Input: part model. Units: mm. Frame: model coordinates. A direction names the side the tool comes from. Coordinates: 2 decimals unless noted, no trailing zeros. Write each loop counter-clockwise with the first axis right and the second up, starting at its lowest first coordinate (ties: lowest second). Pieces come first, ordered by that corner, then holes. Notation, with made-up numbers: (41, 15.25) - (58, 15.25) arc R7 ccw to (58, 22.25) - close; hole circle Ø1 at (61, 88). An arc over 180 degrees is marked (long way). One line per question, with ' | ' between items. Start each with the question number.
1) Draft query along Y for faces 1 (the flat face through (200, 0, 16)), 2 (the flat face through (200, -50.8, 16)), 3 (the flat face through (200, -25, 28.575)), 4 (the flat face through (406.4, -27, 29)). Return one class per face: released by +Y, released by -Y, zero draft, split by the parting line, or undercut.
2) Section query C-C on x = 340.5. Return loops of the section in (y, z) (3 decimals).
3) Section query B-B on z = 9.5. Return loops of the section in (x, y) (3 decimals), and give its area (3 significant figures).
4) Reachability of faces 5 (the flat face through (200, -25, 31.75)), 6 (the flat face through (200, -3.175, 16)) from +Z, -Z, +X, -X, +Y, -Y: full face, straight path, thin tool, end or side. Return the list, or none.
5) First-contact query: P1, Ø1, axis at x = 397.5, z = 2, coming from the +Y side; P2, Ø1.6, axis at y = -20.5, z = 2, coming from the -X side; P3, Ø3.5, axis at y = -32, z = 2.5, coming from the +X side; P4, Ø4, axis at y = -43, z = 25.5, coming from the +X side. Flat tips, straight axial feed; report the tip coordinate or a pass-through.
6) Line query: line 1 (Z direction, x = 285.5, y = -18) (3 decimals); line 2 (Y direction, x = 274.5, z = 26) (3 decimals); line 3 (X direction, y = -16.5, z = 2). Output: solid intervals per line, ascending.
7) Section query A-A on y = -33. Return loops of the section in (x, z) (3 decimals), and give its area (3 significant figures).
```python
from build123d import *

# Parameters (mm, degrees)
F0_W     = 406.4
F0_H     = 31.75
F1_DEPTH = 50.8
F2_T     = -3.175
F3_W     = 19.05
F3_H     = 31.75
F4_DEPTH = 3.175


with BuildPart() as f1:
    # F0 (on Front) → F1 (new body)
    with BuildSketch(Plane.XZ):
        with Locations((203.2, 15.875)):
            Rectangle(F0_W, F0_H)
    extrude(amount=F1_DEPTH)

    # F2
    f2_openings = [f1.faces().sort_by_distance(p)[0] for p in [
        (0, -25.4, 15.875),
        (406.4, -25.4, 15.875),
    ]]
    offset(amount=F2_T, openings=f2_openings)

    # F3 (on face) → F4 (cut)
    with BuildSketch(Plane(origin=(0, 0, 0), x_dir=(1, 0, 0), z_dir=(0, 0, -1))):
        with Locations((9.525, 25.4)):
            Rectangle(F3_W, F3_H)
        with Locations((396.875, 25.4)):
            Rectangle(F3_W, F3_H)
    extrude(amount=-F4_DEPTH, mode=Mode.SUBTRACT)


solid = f1.part
```
Answer key:
1) face 1: released by +Y | face 2: released by -Y | face 3: undercut | face 4: zero draft
2) outline: (-50.8, 0) - (0, 0) - (0, 31.75) - (-50.8, 31.75) - close; hole (-47.625, 3.175) - (-3.175, 3.175) - (-3.175, 28.575) - (-47.625, 28.575) - close
3) outline: (0, -50.8) - (406.4, -50.8) - (406.4, -47.625) - (0, -47.625) - close; (0, -3.175) - (406.4, -3.175) - (406.4, 0) - (0, 0) - close | area: 2,580 mm²
4) face 5: +Z, +X, -X, +Y, -Y | face 6: +X, -X
5) P1: y = 0 | P2: x = 19.05 | P3: x = 387.35 | P4: through
6) line 1: 0 to 3.175, 28.575 to 31.75 | line 2: -50.8 to -47.625, -3.175 to 0 | line 3: 19.05 to 387.35
7) outline: (0, 28.575) - (406.4, 28.575) - (406.4, 31.75) - (0, 31.75) - close; (19.05, 0) - (387.35, 0) - (387.35, 3.175) - (19.05, 3.175) - close | area: 2,460 mm²
